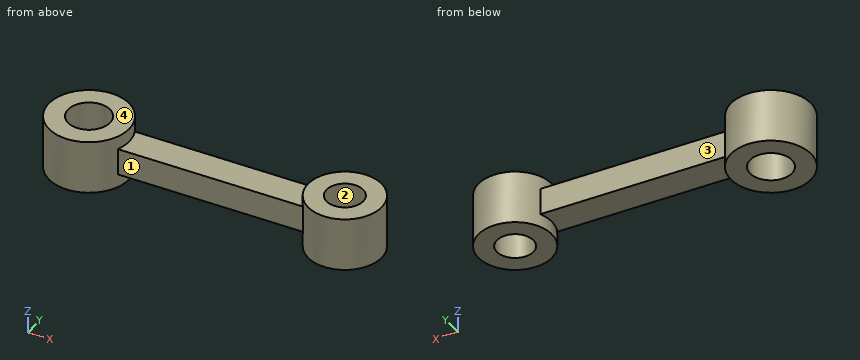
Autodesk Inventor part; units mm, degrees
ref_plane "YZ Plane" through (0, 0, 0) normal (1, 0, 0) x (0, 1, 0)
ref_plane "XZ Plane" through (0, 0, 0) normal (0, 1, 0) x (-1, 0, 0)
ref_plane "XY Plane" through (0, 0, 0) normal (0, 0, 1) x (1, 0, 0)
sketch "Sketch1" plane through (0, 0, 0) normal (0, 0, 1) x (1, 0, 0)
  circle A0 centre (0, 0) radius 3.81
  circle A1 centre (24.13, 0) radius 3.4925
  line L0 (0, 1.4605) -> (24.13, 1.4605)
  line L1 (24.13, 1.4605) -> (24.13, -1.4605)
  line L2 (24.13, -1.4605) -> (0, -1.4605)
  line L3 (0, -1.4605) -> (0, 1.4605)
  dimension "d0" = 7.62
  dimension "d1" = 2.921
  dimension "d2" = 1.4605
  dimension "d3" = 24.13
  dimension "d15" = 6.985
extrude "Extrusion1" add sketch "Sketch1" along normal mid plane 5.08 contours A0 L2 L3 L0 | L0 L3 L2 A0 | L0 L1 L2 A1 | A1 L2 L1 L0
extrude "Extrusion2" add sketch "Sketch1" along normal mid plane 2.54 contours A0 L2 L3 L0 | A0 L0 A1 L2 | L0 L1 L2 A1 picked at (1.27, 0) picked at (22.9658, 0)
hole "Hole2" at (0, 0, 2.54) direction (0, 0, -1) diameter 3.9878 end through all
hole "Hole3" at (24.13, 0, 2.54) direction (0, 0, -1) diameter 3.4798 end through all
equation "\"d2\" = 0.5 * d1"
properties part number "Crank Arm"
Part model, mm, in its own coordinate system. Face numbers are marked on the shaded views. Coordinates: 2 decimals unless noted, no trailing zeros. Loops run counter-clockwise (first coordinate to the right, second up) from the corner with the lowest first, then second, coordinate; pieces in that order, holes last. Notation, with made-up numbers: (-12, 85) - (-4, 85) arc R22 ccw to (-4, 92) - close; hole circle Ø9 at (38, -9). An arc over 180 degrees is marked (long way). Write item = value, one per line. Start each with the question number.
Item 1: Cut at A-A, the plane x = 0. Give the cut face in (y, z), and give its area (3 significant figures).
Item 2: Cut at D-D, the plane y = 0.75. Give the cut face in (x, z).
Item 3: Wall check: L1, parallel to X at y = 0, z = -0.8; L2, parallel to X at y = 0, z = -1.4; L3, parallel to Y at x = 24.13, z = -1.15. Give the ranges that are in metal, low to high. Write a range as from..to.
Item 4: Mould opens along Y. For the marked faces 1, 2, 3 and 4 say: released by +Y, released by -Y, zero draft, split by the parting line, or undercut.
Item 5: Flat gauge pins, fed straight in: pin 1 Ø1.5 at (x, y) = (11, 0) entering from +Z; pin 2 Ø1 at (x, y) = (16, 1) entering from -Z; pin 3 Ø2 at (x, z) = (16, 0.5) entering from +Y. Where does each tip first touch, or does it go through?
Item 6: Cut at C-C, the plane y = -3. Give the cut face in (x, z), and give its area (3 significant figures).
Item 7: Cut at B-B, the plane z = -0.8. Give the cut face in (x, y) (1 decimal).
The answers:
q1.outline = (-3.81, -2.54) - (-1.99, -2.54) - (-1.99, 2.54) - (-3.81, 2.54) - close; (1.99, -2.54) - (3.81, -2.54) - (3.81, 2.54) - (1.99, 2.54) - close
q1.area = 18.5 mm2
q2.outline = (-3.74, -2.54) - (-1.85, -2.54) - (-1.85, 2.54) - (-3.74, 2.54) - close; (1.85, -2.54) - (3.74, -2.54) - (3.74, -1.27) - (20.72, -1.27) - (20.72, -2.54) - (22.56, -2.54) - (22.56, 2.54) - (20.72, 2.54) - (20.72, 1.27) - (3.74, 1.27) - (3.74, 2.54) - (1.85, 2.54) - close; (25.7, -2.54) - (27.54, -2.54) - (27.54, 2.54) - (25.7, 2.54) - close
q3.L1 = -3.81..-1.99, 1.99..22.39, 25.87..27.62
q3.L2 = -3.81..-1.99, 1.99..3.81, 20.64..22.39, 25.87..27.62
q3.L3 = -3.49..-1.74, 1.74..3.49
q4.face_1 = released by -Y
q4.face_2 = undercut
q4.face_3 = released by +Y
q4.face_4 = zero draft
q5.pin_1 = 1.27
q5.pin_2 = -1.27
q5.pin_3 = 1.46
q6.outline = (-2.35, -2.54) - (2.35, -2.54) - (2.35, 2.54) - (-2.35, 2.54) - close; (22.34, -2.54) - (25.92, -2.54) - (25.92, 2.54) - (22.34, 2.54) - close
q6.area = 42.0 mm2
q7.outline = (3.5, -1.5) - (21, -1.5) arc R3.5 ccw (long way) to (21, 1.5) - (3.5, 1.5) arc R3.8 ccw (long way) to start; hole circle Ø4 at (0, 0); hole circle Ø3.5 at (24.1, 0)
